from build123d import *

# Parameters (mm, degrees)
SKETCH1_W           = 110
SKETCH1_H           = 70
BOSS_EXTRUDE1_DEPTH = 10
SKETCH5_R           = 1.9
CUT_EXTRUDE4_DEPTH  = 77.548290163
CUT_EXTRUDE6_DEPTH  = 6
SKETCH17_R          = 1.9
CUT_EXTRUDE8_DEPTH  = 77.548290163
FILLET1_R           = 2
SKETCH24_R          = 1.9
CUT_EXTRUDE12_DEPTH = 77.548290163
SKETCH25_R          = 1.9
CUT_EXTRUDE13_DEPTH = 77.548290163
CUT_EXTRUDE15_DEPTH = 6
CUT_EXTRUDE16_DEPTH = 6
CUT_EXTRUDE17_DEPTH = 6
CUT_EXTRUDE18_DEPTH = 6


with BuildPart() as part:
    # Sketch1 → Boss-Extrude1 (new body)
    with BuildSketch(Plane(origin=(0, 0, 0), x_dir=(1, 0, 0), z_dir=(0, 1, 0))):
        with Locations((9.869408673, 4.390361071)):
            Rectangle(SKETCH1_W, SKETCH1_H)
    extrude(amount=BOSS_EXTRUDE1_DEPTH)

    # Sketch5 → Cut-Extrude4 (cut, through all)
    with BuildSketch(Plane(origin=(0, 10, 0), x_dir=(1, 0, 0), z_dir=(0, 1, 0))):
        with Locations(Location((9.869408673, -20.609638929, 0), (0, 0, 270))):
            Circle(SKETCH5_R)
    extrude(amount=-CUT_EXTRUDE4_DEPTH, mode=Mode.SUBTRACT)

    # Sketch14 → Cut-Extrude6 (cut)
    with BuildSketch(Plane.XY.offset(30.609638929)):
        Polygon((-45.130591327, 0), (-45.130591327, 4), (64.869408673, 2), (64.869408673, 0), align=None)
    extrude(amount=-CUT_EXTRUDE6_DEPTH, mode=Mode.SUBTRACT)

    # Sketch17 → Cut-Extrude8 (cut, through all)
    with BuildSketch(Plane(origin=(0, 0, 0), x_dir=(-1, 0, 0), z_dir=(0, -1, 0))):
        with Locations(Location((-9.869408673, 30.128732458, 0), (0, 0, 90))):
            Circle(SKETCH17_R)
    extrude(amount=-CUT_EXTRUDE8_DEPTH, mode=Mode.SUBTRACT)

    # Fillet1
    fillet1_edges = [part.edges().sort_by_distance(p)[0] for p in [
        (9.869408673, 3, 24.609638929),
    ]]
    fillet(fillet1_edges, radius=FILLET1_R)

    # Sketch24 → Cut-Extrude12 (cut, through all)
    with BuildSketch(Plane.XZ):
        with Locations(Location((44.869408673, 5.609638929, 0), (0, 0, 270))):
            Circle(SKETCH24_R)
    extrude(amount=-CUT_EXTRUDE12_DEPTH, mode=Mode.SUBTRACT)

    # Sketch25 → Cut-Extrude13 (cut, through all)
    with BuildSketch(Plane.XZ):
        with Locations(Location((-25.130591327, -14.390361071, 0), (0, 0, 270))):
            Circle(SKETCH25_R)
    extrude(amount=-CUT_EXTRUDE13_DEPTH, mode=Mode.SUBTRACT)

    # Sketch27 → Cut-Extrude15 (cut)
    with BuildSketch(Plane(origin=(0, 10, 0), x_dir=(1, 0, 0), z_dir=(0, 1, 0))):
        Polygon((14.369408673, 30.128732458), (12.119408673, 34.025846775), (7.619408673, 34.025846775), (5.369408673, 30.128732458), (7.619408673, 26.231618141), (12.119408673, 26.231618141), align=None)
    extrude(amount=-CUT_EXTRUDE15_DEPTH, mode=Mode.SUBTRACT)

    # Sketch30 → Cut-Extrude16 (cut)
    with BuildSketch(Plane(origin=(0, 10, 0), x_dir=(1, 0, 0), z_dir=(0, 1, 0))):
        Polygon((49.369408673, -5.609638929), (47.119408673, -1.712524612), (42.619408673, -1.712524612), (40.369408673, -5.609638929), (42.619408673, -9.506753246), (47.119408673, -9.506753246), align=None)
    extrude(amount=-CUT_EXTRUDE16_DEPTH, mode=Mode.SUBTRACT)

    # Sketch31 → Cut-Extrude17 (cut)
    with BuildSketch(Plane(origin=(0, 10, 0), x_dir=(1, 0, 0), z_dir=(0, 1, 0))):
        Polygon((14.369408673, -20.609638929), (12.119408673, -16.712524612), (7.619408673, -16.712524612), (5.369408673, -20.609638929), (7.619408673, -24.506753246), (12.119408673, -24.506753246), align=None)
    extrude(amount=-CUT_EXTRUDE17_DEPTH, mode=Mode.SUBTRACT)

    # Sketch32 → Cut-Extrude18 (cut)
    with BuildSketch(Plane(origin=(0, 10, 0), x_dir=(1, 0, 0), z_dir=(0, 1, 0))):
        Polygon((-20.630591327, 14.390361071), (-22.880591327, 18.287475388), (-27.380591327, 18.287475388), (-29.630591327, 14.390361071), (-27.380591327, 10.493246754), (-22.880591327, 10.493246754), align=None)
    extrude(amount=-CUT_EXTRUDE18_DEPTH, mode=Mode.SUBTRACT)


solid = part.part
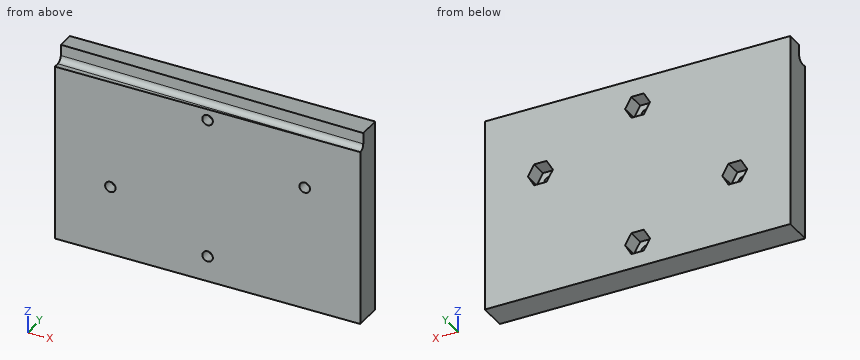
Could you check a few things on this model? Use its own coordinates, in mm. Give positions to 0.01 mm unless a question says otherwise; leave off trailing zeros. Order: outer loops, then holes, each group sorted by start corner. A loop starts at its lowest first (then second) coordinate and runs counter-clockwise, first axis right, second up.
1. Will this pin go through, and if not, where does the flat tip stop? P1, Ø5, axis at x = 9.87, z = -30.13, coming from the +Y side.
2. Suppose I cut it at A-A (y = 8). List the corners of the cut face in (x, z) for me.
3. I need wall thicknesses on L1, parallel to Z at x = 12, y = 7; L2, parallel to Z at x = 46, y = 5.25; L3, parallel to Y at x = 12, z = 17.5. Which ranges of each line are inside material? Lowest first, please.
Solved:
1. P1: stops at y = 4
2. outline: (-45.13, -39.39) - (64.87, -39.39) - (64.87, 30.61) - (-45.13, 30.61) - close; hole (-29.63, -14.39) - (-27.38, -18.29) - (-22.88, -18.29) - (-20.63, -14.39) - (-22.88, -10.49) - (-27.38, -10.49) - close; hole (5.37, -30.13) - (7.62, -34.03) - (12.12, -34.03) - (14.37, -30.13) - (12.12, -26.23) - (7.62, -26.23) - close; hole (5.37, 20.61) - (7.62, 16.71) - (12.12, 16.71) - (14.37, 20.61) - (12.12, 24.51) - (7.62, 24.51) - close; hole (40.37, 5.61) - (42.62, 1.71) - (47.12, 1.71) - (49.37, 5.61) - (47.12, 9.51) - (42.62, 9.51) - close
3. L1: z = -39.39 to -34.03, -26.23 to 16.71, 24.51 to 30.61
3. L2: z = -39.39 to 1.71, 9.51 to 30.61
3. L3: y = 0 to 4
